Read the model definition and answer for the solid it produces. Units are mm, in the model's axes. Face numbers are marked on the shaded views. A direction names the side the tool comes from. Give positions to 0.01 mm unless a question says otherwise; leave off trailing zeros. Loops run counter-clockwise (first coordinate to the right, second up) from the corner with the lowest first, then second, coordinate; pieces in that order, holes last. Notation, with made-up numbers: (72.25, -11.75) - (111.25, -11.75) arc R24 cw to (111.25, 15.25) - close; hole circle Ø5 at (34, 62). An arc over 180 degrees is marked (long way). Write each question's results on one line, items separated by ' | '. Start each with the question number.
Q1. Given pin 1 (6 mm diameter, centred on y = -10.5, z = 6, fed in from -X); pin 2 (22 mm diameter, centred on y = 5.5, z = 13, fed in from +X); pin 3 (10 mm diameter, centred on x = -15, y = 8.5, fed in from +Z), each flat-ended and moving along its own axis, determine where each tip first touches the part or whether it passes through.
Q2. Find the intervals of material crossed by line 1 (Y direction, x = 0, z = -1); line 2 (Y direction, x = -8, z = 19.55); line 3 (X direction, y = -18, z = 20.6), in increasing order. Write a range as from..to.
Q3. For the marked faces 4, 5, 6, 7 and 8, determine the directions among +Z, -Z, +X, -X, +Y, -Y from which every point of the face is accessible in a straight line to the end or side of a thin tool.
Q4. The part is cut by section C-C, the plane z = -9. Write down the section's boundary in (x, y).
Q5. Determine the mould class of the marked faces 1, 2 and 3 for opening direction X: +X half, -X half, draft (parallel to the pull), parting line (faces both ways), or undercut.
Q6. The part is cut by section B-B, the plane y = -39. Write down the section's boundary in (x, z).
Q7. The part is cut by section A-A, the plane x = 0. State how many separate pieces and enclosed holes the cut face has, plus the area to 3 significant figures.
```python
from build123d import *
from build123d.topology import SkipClean

# Parameters (mm, degrees)
SKETCH_1_W           = 120
SKETCH_1_H           = 60
EXTRUDE_1_DEPTH      = 47
SHELL_2_T            = -3
SKETCH_2_W           = 55
SKETCH_2_H           = 41
CUT_EXTRUDE_1_DEPTH  = 3
SKETCH_5_W           = 88
SKETCH_5_H           = 41
CUT_EXTRUDE_3_DEPTH  = 10
SKETCH_6_R           = 2.5
CUT_EXTRUDE_4_DEPTH  = 82.908485519
EXTRUDE_4_REACH      = 82.225
CUT_EXTRUDE_5_REACH  = 83.908
SKETCH_9_W           = 17
SKETCH_9_H           = 25
SKETCH_10_R          = 1.6
EXTRUDE_5_DEPTH      = 18
SKETCH_13_W          = 33
SKETCH_13_H          = 29
SKETCH_13_W_2        = 29
SKETCH_13_H_2        = 25
EXTRUDE_6_DEPTH      = 2
SKETCH_14_W          = 10
SKETCH_14_H          = 16
SKETCH_14_R          = 1.75
EXTRUDE_7_DEPTH      = 22
SKETCH_15_R          = 10.5
CUT_EXTRUDE_7_DEPTH  = 12
CUT_EXTRUDE_8_DEPTH  = 6
SKETCH_19_W          = 34
SKETCH_19_H          = 16
CUT_EXTRUDE_9_DEPTH  = 18
SKETCH_16_W          = 1
SKETCH_16_H          = 16
SKETCH_16_W_2        = 11
SKETCH_16_H_2        = 2
EXTRUDE_8_DEPTH      = 22
SKETCH_20_W          = 6
SKETCH_20_H          = 6
CUT_EXTRUDE_10_DEPTH = 11
SKETCH_21_W          = 120
SKETCH_21_H          = 3
EXTRUDE_9_DEPTH      = 14
SKETCH_11_R          = 1.75
CUT_EXTRUDE_6_DEPTH  = 89.005681635


with BuildPart() as part:
    # 草图1 → 凸台-拉伸1 (new body)
    with BuildSketch(Plane(origin=(0, 0, 0), x_dir=(1, 0, 0), z_dir=(0, 0, -1))):
        Rectangle(SKETCH_1_W, SKETCH_1_H)
    extrude(amount=EXTRUDE_1_DEPTH)

    # 抽壳2
    shell_2_openings = [part.faces().sort_by_distance(p)[0] for p in [
        (60, 0, -23.5),
        (-60, 0, -23.5),
    ]]
    offset(amount=SHELL_2_T, openings=shell_2_openings, kind=Kind.INTERSECTION)

    # 草图2 → 切除-拉伸1 (cut)
    with BuildSketch(Plane(origin=(0, 30, 45), x_dir=(-1, 0, 0), z_dir=(0, -1, 0))):
        with Locations((0, 68.5)):
            Rectangle(SKETCH_2_W, SKETCH_2_H)
    extrude(amount=CUT_EXTRUDE_1_DEPTH, mode=Mode.SUBTRACT)

    # 草图5 → 切除-拉伸3 (cut)
    with BuildSketch(Plane.XZ.offset(30)):
        with Locations((0, -23.5)):
            Rectangle(SKETCH_5_W, SKETCH_5_H)
    extrude(amount=-CUT_EXTRUDE_3_DEPTH, mode=Mode.SUBTRACT)

    # 草图6 → 切除-拉伸4 (cut, through all)
    with BuildSketch(Plane.XY):
        with Locations((0, -18)):
            Circle(SKETCH_6_R)
    extrude(amount=-CUT_EXTRUDE_4_DEPTH, mode=Mode.SUBTRACT)

    # 草图8 → 凸台-拉伸4 (add, up to next)
    with BuildSketch(Plane(origin=(0, 0, -44), x_dir=(-1, 0, 0), z_dir=(0, 0, -1)), mode=Mode.PRIVATE) as extrude_4_sk1:
        Polygon((-60, -27), (-44, -25.270549885), (-44, -30), (-60, -30), align=None)
    extrude_4_tool1 = extrude(extrude_4_sk1.sketch, amount=-EXTRUDE_4_REACH, mode=Mode.PRIVATE) - part.part
    extrude_4 = extrude_4_tool1.solids().sort_by_distance((51.403338, -28.035391, -44))[0]
    add(extrude_4)

    # 镜向1: 凸台-拉伸4 across plane
    add(extrude_4.mirror(Plane(origin=(0, 0, 0), x_dir=(0, 0, 1), z_dir=(1, 0, 0))))

    # 草图9 → 切除-拉伸5 (cut, up to next)
    with BuildSketch(Plane.XY, mode=Mode.PRIVATE) as cut_extrude_5_sk1:
        with Locations((0, 6.5)):
            Rectangle(SKETCH_9_W, SKETCH_9_H)
    cut_extrude_5_tool1 = extrude(cut_extrude_5_sk1.sketch, amount=-CUT_EXTRUDE_5_REACH, mode=Mode.PRIVATE) & part.part
    add(cut_extrude_5_tool1.solids().sort_by_distance((0, 6.5, 0))[0], mode=Mode.SUBTRACT)

    # 草图10 → 凸台-拉伸5 (add)
    with BuildSketch(Plane.XY):
        Polygon((-10.5, -8), (10.5, -8), (16.5, -8), (16.5, 21), (-16.5, 21), (-16.5, -8), align=None)
        with Locations((-12.5, 6.5)):
            Circle(SKETCH_10_R, mode=Mode.SUBTRACT)
        with Locations((12.5, 6.5)):
            Circle(SKETCH_10_R, mode=Mode.SUBTRACT)
        Polygon((-8.5, 11), (14.5, 11), (14.5, 19), (-14.5, 19), (-14.5, 11), align=None, mode=Mode.SUBTRACT)
        Polygon((-8.5, 9.8), (8.5, 9.8), (8.5, 2.5), (14.5, 2.5), (14.5, -6), (-14.5, -6), (-14.5, 2.5), (-8.5, 2.5), align=None, mode=Mode.SUBTRACT)
    extrude(amount=EXTRUDE_5_DEPTH)

    # 草图13 → 凸台-拉伸6 (add)
    with BuildSketch(Plane.XY.offset(18)):
        with Locations((0, 6.5)):
            Rectangle(SKETCH_13_W, SKETCH_13_H)
        with Locations((0, 6.5)):
            Rectangle(SKETCH_13_W_2, SKETCH_13_H_2, mode=Mode.SUBTRACT)
    extrude(amount=EXTRUDE_6_DEPTH)

    # 草图14 → 凸台-拉伸7 (add)
    # profile 1 of 2: a face of its own
    with BuildSketch(Plane.XY):
        with Locations((-10.5, -16)):
            Rectangle(SKETCH_14_W, SKETCH_14_H)
        with Locations((-8, -18)):
            Circle(SKETCH_14_R, mode=Mode.SUBTRACT)
    # profile 2 of 2: a face of its own
    with BuildSketch(Plane.XY):
        with Locations((22.5, -16)):
            Rectangle(SKETCH_14_W, SKETCH_14_H)
        with Locations((20, -18)):
            Circle(SKETCH_14_R, mode=Mode.SUBTRACT)
    extrude(amount=EXTRUDE_7_DEPTH)

    # 草图15 → 切除-拉伸7 (cut)
    with BuildSketch(Plane.XY):
        with Locations((0, -18)):
            Circle(SKETCH_15_R)
    extrude(amount=CUT_EXTRUDE_7_DEPTH, mode=Mode.SUBTRACT)

    # 草图17 → 切除-拉伸8 (cut)
    with SkipClean():  # the faces are left unmerged after this step: merging them gives an invalid solid
        with BuildSketch(Plane(origin=(0, 0, 12), x_dir=(-1, 0, 0), z_dir=(0, 0, -1))):
            with BuildLine():
                Line((5.5, -9.05572809), (5.5, -24))
                Line((5.5, -24), (8.61684397, -24))
                ThreePointArc((8.61684397, -24), (10.278819808, -15.856203519), (5.5, -9.05572809))
            make_face()
        extrude(amount=-CUT_EXTRUDE_8_DEPTH, mode=Mode.SUBTRACT)

    # 草图19 → 切除-拉伸9 (cut)
    with BuildSketch(Plane.XY):
        with Locations((6, -16)):
            Rectangle(SKETCH_19_W, SKETCH_19_H)
    extrude(amount=CUT_EXTRUDE_9_DEPTH, mode=Mode.SUBTRACT)

    # 草图16 → 凸台-拉伸8 (add)
    with BuildSketch(Plane.XY):
        with Locations((-16, -16)):
            Rectangle(SKETCH_16_W, SKETCH_16_H)
        with Locations((22, -7)):
            Rectangle(SKETCH_16_W_2, SKETCH_16_H_2)
    extrude(amount=EXTRUDE_8_DEPTH)

    # 草图20 → 切除-拉伸10 (cut)
    with BuildSketch(Plane(origin=(0, 0, -3), x_dir=(-1, 0, 0), z_dir=(0, 0, -1))):
        with Locations((-12.5, 6.5)):
            Rectangle(SKETCH_20_W, SKETCH_20_H)
        with Locations((12.5, 6.5)):
            Rectangle(SKETCH_20_W, SKETCH_20_H)
    extrude(amount=-CUT_EXTRUDE_10_DEPTH, mode=Mode.SUBTRACT)

    # 草图21 → 凸台-拉伸9 (add)
    with BuildSketch(Plane.XZ.offset(30)):
        with Locations((0, -1.5)):
            Rectangle(SKETCH_21_W, SKETCH_21_H)
    extrude(amount=EXTRUDE_9_DEPTH)

    # 草图11 → 切除-拉伸6 (cut, through all)
    with BuildSketch(Plane(origin=(0, 0, 0), x_dir=(-1, 0, 0), z_dir=(0, 0, -1))):
        with Locations(Location((-50, 20, 0), (0, 0, 180))):
            Circle(SKETCH_11_R)
        with Locations(Location((50, 20, 0), (0, 0, 180))):
            Circle(SKETCH_11_R)
        with Locations(Location((-50, -39, 0), (0, 0, 180))):
            Circle(SKETCH_11_R)
        with Locations(Location((50, -39, 0), (0, 0, 180))):
            Circle(SKETCH_11_R)
    extrude(amount=CUT_EXTRUDE_6_DEPTH, mode=Mode.SUBTRACT)


solid = part.part
```
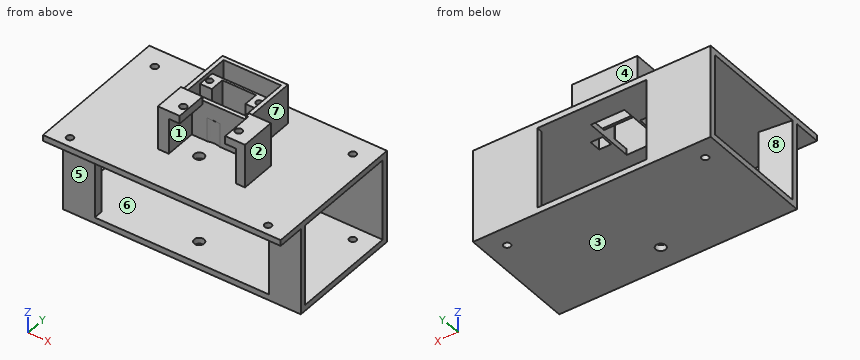
Check sheet entries:
1) pin 1: stops at x = -16.5 | pin 2: stops at x = 16.5 | pin 3: stops at z = 20
2) line 1: y = -44..-20.5, -15.5..-6, 19..30 | line 2: y = -24..-19.75, -16.25..-6, 19..21 | line 3: x = -16.5..-9.75, -6.25..-5.5, 17.5..18.25, 21.75..27.5
3) face 4: +Z, +X, -X, +Y | face 5: -Z, +X, -X, -Y | face 6: none | face 7: +Z, +X, +Y | face 8: -X
4) outline: (-60, -30) - (-44, -30) - (-44, -25.27) - (-60, -27) - close; (-60, 27) - (-27.5, 27) - (-27.5, 30) - (-60, 30) - close; (27.5, 27) - (60, 27) - (60, 30) - (27.5, 30) - close; (44, -30) - (60, -30) - (60, -27) - (44, -25.27) - close
5) face 1: undercut | face 2: +X half | face 3: draft
6) outline: (-60, -3) - (-51.75, -3) - (-51.75, 0) - (-60, 0) - close; (-48.25, -3) - (48.25, -3) - (48.25, 0) - (-48.25, 0) - close; (51.75, -3) - (60, -3) - (60, 0) - (51.75, 0) - close
7) separate pieces: 6 | enclosed holes: 0 | area: 393 mm^2
